Source: CAD feature listing. Evaluate the final solid. Frame: model axes, mm. Face numbers are marked on the shaded views. A direction names the side the tool comes from. Give positions to 0.01 mm unless a question says otherwise; leave off trailing zeros. Write each loop counter-clockwise with the first axis right and the second up, starting at its lowest first coordinate (ties: lowest second). Pieces come first, ordered by that corner, then holes. Notation, with made-up numbers: (86.25, 69.25) -> (133.25, 69.25) arc R20 ccw to (133.25, 82.25) -> close; hole circle Ø8 at (37, -8.75). An arc over 180 degrees is marked (long way). Use one line per item in the form item = value. Start each with the question number.
(1) Cut plane B-B, the plane z = 16.25. Output: boundary loops of the cut face in (x, y).
(2) Cut plane C-C, the plane y = 8. Output: boundary loops of the cut face in (x, z).
(3) Cut plane A-A, the plane y = 0. Output: boundary loops of the cut face in (x, z), and give its area (3 significant figures).
(4) Material intervals for line 1 along X through (y, z) = (-4.5, 9.5); line 2 along Z through (x, y) = (7.25, -10.5); line 3 along Y through (x, z) = (18, 8), sorted ascending. Write a range as from..to.
(5) First-contact query: P1, Ø2.5, axis at x = 21.5, z = 8, coming from the -Y side; P2, Ø9.5, axis at x = 4.5, y = 0.5, coming from the +Z side; P3, Ø4, axis at x = 5.5, y = 9.5, coming from the +Z side (3 decimals). Flat tips, straight axial feed; report the tip coordinate or a pass-through.
(6) Cut plane D-D, the plane x = 10.5. Output: boundary loops of the cut face in (y, z) (3 decimals).
(7) Set-up query: the marked faces 1 and 2. Return all of +Z, -Z, +X, -X, +Y, -Y with unobstructed straight access to the full face (end or side cutting, diameter ignored); none if empty.
from build123d import *

# Parameters (mm, degrees)
F1_DEPTH = 19.05
F3_DEPTH = 25.401
F5_DEPTH = 12.7


with BuildPart() as f1:
    # F0 (on Front) → F1 (new body, symmetric)
    with BuildSketch(Plane.XZ):
        Polygon((0, 6.35), (0, 0), (25.4, 0), (25.4, 6.35), (16.9333333333, 6.35), align=None)
        Polygon((0, 20.6375), (0, 6.35), (16.9333333333, 6.35), (16.9333333333, 12.7), (6.35, 20.6375), align=None)
        Polygon((16.9333333333, 6.35), (25.4, 6.35), (16.9333333333, 12.7), align=None)
        Polygon((0, 25.4), (0, 20.6375), (6.35, 20.6375), align=None)
    extrude(amount=F1_DEPTH, both=True)

    # F2 (on face) → F3 (cut, through all)
    with BuildSketch(Plane(origin=(0, 0, 0), x_dir=(0, -1, 0), z_dir=(-1, 0, 0))):
        Polygon((6.35, 6.35), (19.05, 6.35), (19.05, 25.4), (-6.35, 25.4), (-6.35, 19.05), (6.35, 19.05), align=None)
    extrude(amount=-F3_DEPTH, mode=Mode.SUBTRACT)

    # F4 (on face) → F5 (cut)
    with BuildSketch(Plane.XZ.offset(6.35)):
        Polygon((19.05, 6.35), (25.4, 6.35), (19.05, 11.1125), align=None)
    extrude(amount=-F5_DEPTH, mode=Mode.SUBTRACT)


solid = f1.part
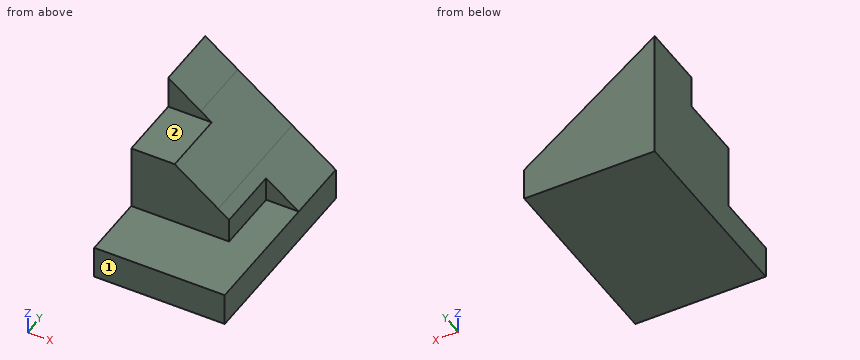
Geometry says:
q1.outline = (0, -6.35) -> (12.2, -6.35) -> (12.2, 19.05) -> (0, 19.05) -> close
q2.outline = (0, 0) -> (25.4, 0) -> (25.4, 6.35) -> (0, 25.4) -> close
q3.outline = (0, 0) -> (25.4, 0) -> (25.4, 6.35) -> (19.05, 6.35) -> (19.05, 11.11) -> (8.47, 19.05) -> (0, 19.05) -> close
q3.area = 361 mm^2
q4.line_1 = 0..19.05
q4.line_2 = 0..6.35
q4.line_3 = -6.35..19.05
q5.P1 = 6.35
q5.P2 = 19.05
q5.P3 = 22.775
q6.outline = (-19.05, 0) -> (19.05, 0) -> (19.05, 17.525) -> (-6.35, 17.525) -> (-6.35, 6.35) -> (-19.05, 6.35) -> close
q7.face_1 = +Z, -Z, +X, -X, -Y
q7.face_2 = +Z, +X, -X, -Y
